Part model, mm, in its own coordinate system. Face numbers are marked on the shaded views. Give positions to 0.01 mm unless a question says otherwise; leave off trailing zeros. Order: outer loops, then holes, each group sorted by start corner. A loop starts at its lowest first (then second) coordinate and runs counter-clockwise, first axis right, second up. Notation, with made-up numbers: M -28,58.5 L -6,58.5 A8 cw -6,71.5 Z; hole C 67,19 d4. An arc over 180 degrees is marked long. One line per question, with ' | ' between items.
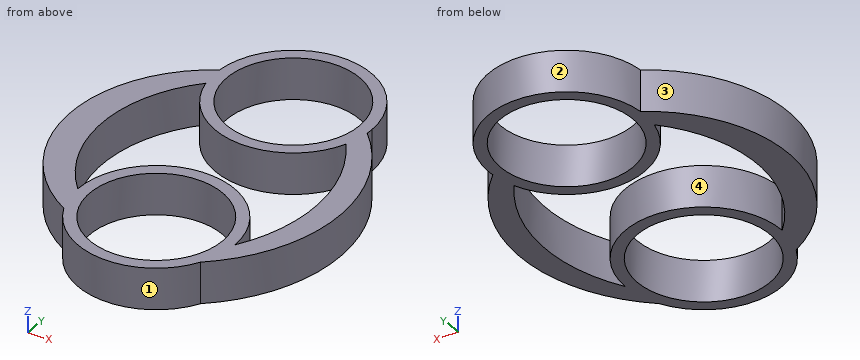
```python
from build123d import *

# Parameters (mm, degrees)
F0_R     = 11.2
F1_DEPTH = 7


with BuildPart() as f1:
    # F0 (on Top) → F1 (new body)
    with BuildSketch(Plane.XY):
        with BuildLine():
            ThreePointArc((11.59233, -6.31331), (12.79177, -3.257395), (13.2, 0))
            ThreePointArc((13.2, 0), (0, 13.2), (-13.2, 0))
            ThreePointArc((-13.2, 0), (-12.920509, -2.701933), (-12.093872, -5.289448))
            ThreePointArc((-12.093872, -5.289448), (-0.570052, -13.187685), (11.59233, -6.31331))
        make_face()
        Circle(F0_R, mode=Mode.SUBTRACT)
        with BuildLine():
            ThreePointArc((12.173578, 30.230427), (17.326701, 15.272754), (13.2, 0))
            ThreePointArc((13.2, 0), (12.79177, -3.257395), (11.59233, -6.31331))
            ThreePointArc((11.59233, -6.31331), (21.438452, 13.603178), (13.152736, 34.217724))
            ThreePointArc((13.152736, 34.217724), (12.819133, 32.185772), (12.173578, 30.230427))
        make_face()
        with BuildLine():
            ThreePointArc((-12.093872, -5.289448), (-12.920509, -2.701933), (-13.2, 0))
            ThreePointArc((-13.2, 0), (-19.597353, 16.33302), (-12.902327, 32.546295))
            ThreePointArc((-12.902327, 32.546295), (-13.174098, 34.507228), (-13.149548, 36.486753))
            ThreePointArc((-13.149548, 36.486753), (-24.758622, 15.291955), (-12.093872, -5.289448))
        make_face()
        with BuildLine():
            ThreePointArc((-12.902327, 32.546295), (-1.213911, 22.189696), (12.173578, 30.230427))
            ThreePointArc((12.173578, 30.230427), (12.819133, 32.185772), (13.152736, 34.217724))
            ThreePointArc((13.152736, 34.217724), (13.188179, 34.775242), (13.2, 35.33376))
            ThreePointArc((13.2, 35.33376), (0.577048, 48.521141), (-13.149548, 36.486753))
            ThreePointArc((-13.149548, 36.486753), (-13.174098, 34.507228), (-12.902327, 32.546295))
        make_face()
        with Locations((0, 35.33376)):
            Circle(F0_R, mode=Mode.SUBTRACT)
    extrude(amount=F1_DEPTH)


solid = f1.part
```
1. Slice it at C-C on y = -3. Give the cut face in (x, z), then the cut area to 3 significant figures.
Worked out:
outline: M -15.59,0 L -10.79,0 L -10.79,7 L -15.59,7 Z; M 10.79,0 L 14.96,0 L 14.96,7 L 10.79,7 Z | area: 62.7 mm2
2. Mould opens along Y. For the marked faces 1, 2, 3 and 4 say: released by +Y, released by -Y, zero draft, split by the parting line, or undercut.
Worked out:
face 1: released by -Y | face 2: released by +Y | face 3: split by the parting line | face 4: undercut
3. Probe L1, parallel to Y at x = 0, z = 2.75; L2, parallel to X at y = 27.5, z = 4.75; L3, parallel to X at y = 5, z = 5.5. List the from-to ranges inside material, lowest first. Write a range as from..to.
Worked out:
L1: y = -13.2..-11.2, 11.2..13.2, 22.13..24.13, 46.53..48.53 | L2: x = -21.78..-16.66, -10.62..-8, 8..10.62, 13.92..18.23 | L3: x = -22.15..-16.8, -12.22..-10.02, 10.02..12.22, 15.67..19.69
4. Drop flat-ended pins along their axis: pin 1 (4 mm diameter, centred on x = -4, z = 6.5, fed in from +Y); pin 2 (10 mm diameter, centred on x = -5.5, y = 10, fed in from -Z); pin 3 (4 mm diameter, centred on x = -19, z = 4.5, fed in from -Y); pin 4 (2 mm diameter, centred on y = 13.5, z = 1, fed in from -X). Give the stop position or say it passes through.
Worked out:
pin 1: stops at y = 48.38 | pin 2: stops at z = 0 | pin 3: stops at y = -1.8 | pin 4: stops at x = -24.73
5. Slice it at A-A on z = 1.25. Give the cut face in (x, y), then the cut area to 3 significant figures.
Worked out:
outline: M -13.15,36.49 A24.05 ccw -12.09,-5.29 A13.2 ccw 11.59,-6.31 A27.2 ccw 13.15,34.22 A13.2 ccw 13.2,35.33 A13.2 ccw Z; hole M -13.2,0 A13.2 cw 13.2,0 A26.96 ccw 12.17,30.23 A13.2 cw -12.9,32.55 A23.5 ccw Z; hole C 0,0 d22.4; hole C 0,35.33 d22.4 | area: 650 mm2
6. Slice it at D-D on x = 14. Give the cut face in (y, z).
Worked out:
outline: M -4.06,0 L 1.36,0 L 1.36,7 L -4.06,7 Z; M 27.36,0 L 33.36,0 L 33.36,7 L 27.36,7 Z
7. Slice it at B-B on x = 0. Give the cut face in (y, z), then the cut area to 3 significant figures.
Worked out:
outline: M -13.2,0 L -11.2,0 L -11.2,7 L -13.2,7 Z; M 11.2,0 L 13.2,0 L 13.2,7 L 11.2,7 Z; M 22.13,0 L 24.13,0 L 24.13,7 L 22.13,7 Z; M 46.53,0 L 48.53,0 L 48.53,7 L 46.53,7 Z | area: 56.0 mm2
